Geometry: see drawing. Coordinates: mm, zero at the bounding-box minimum. Give positions to 0.01 mm unless a question says otherwise; leave off trailing zeros. Write each loop counter-clockwise with the first axis right and the second up, starting at its lowest first coordinate (ties: lowest second). Pieces come first, ordered by that corner, then holes. Notation, with made-up numbers: (-33.5, -38.5) - (-19.5, -38.5) arc R20 cw to (-19.5, -24.5) - close; hole circle Ø9 at (-12.75, 51). An arc over 180 degrees is marked (long way). Use a Markdown table: item, result. Add a question column.
1. Section query A-A, the plane z = 1.9. Return loops of the section in (x, y).
2. Section query C-C, the plane y = 61. Return loops of the section in (x, z).
3. Section query B-B, the plane x = 36.5. Return loops of the section in (y, z), plus the area to 3 significant figures.
4. Material intervals for probe 1 along X at (y, z) = (59.5, 0.9); probe 2 along Y at (x, z) = (38, 0.7); probe 3 along X at (y, z) = (38, 2.95), sorted ascending.
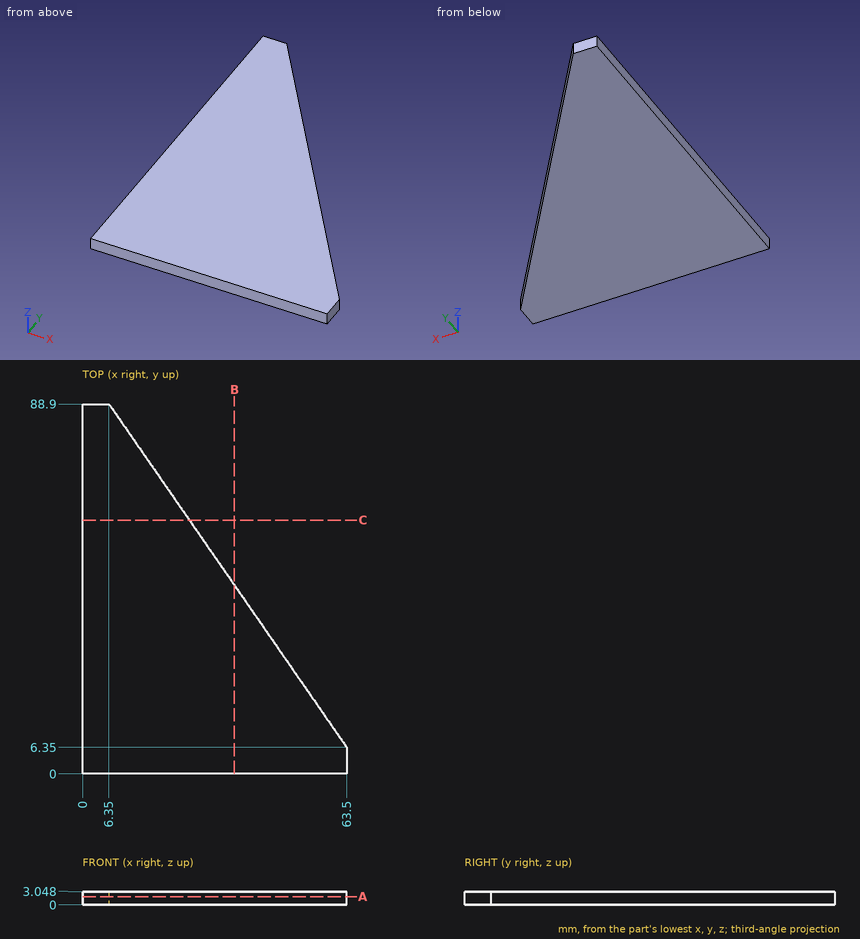
Result sheet:
| question | item | result |
|---|---|---|
| 1 | outline | (0, 0) - (63.5, 0) - (63.5, 6.35) - (6.35, 88.9) - (0, 88.9) - close |
| 2 | outline | (0, 0) - (25.67, 0) - (25.67, 3.05) - (0, 3.05) - close |
| 3 | outline | (0, 0) - (45.35, 0) - (45.35, 3.05) - (0, 3.05) - close |
| 3 | area | 138 mm² |
| 4 | probe 1 | x = 0 to 26.7 |
| 4 | probe 2 | y = 0 to 43.18 |
| 4 | probe 3 | x = 0 to 41.59 |
